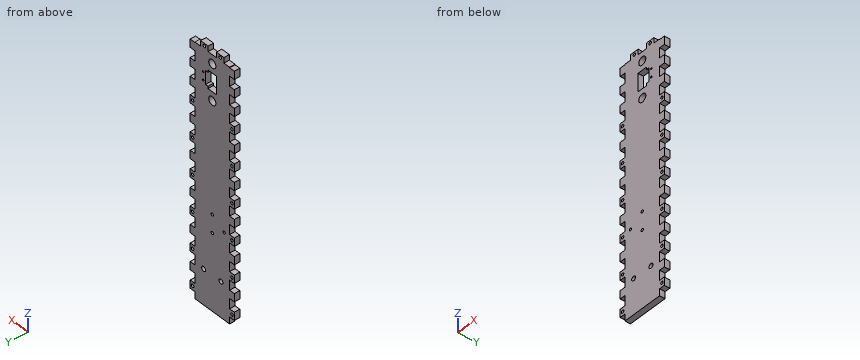
from build123d import *

# Parameters (mm, degrees)
SKETCH1_W               = 44
SKETCH1_H               = 6
BOSS_EXTRUDE1_DEPTH     = 277
SKETCH4_W               = 9
SKETCH4_H               = 6
BOSS_EXTRUDE2_DEPTH     = 6
SKETCH5_W               = 9
SKETCH5_H               = 6
BOSS_EXTRUDE3_DEPTH     = 6
SKETCH6_W               = 9.5
SKETCH6_H               = 6
BOSS_EXTRUDE4_DEPTH     = 6
SKETCH7_R               = 1.6
CUT_EXTRUDE1_DEPTH      = 286.346184868
SKETCH8_R               = 2.5
CUT_EXTRUDE2_DEPTH      = 12
SKETCH9_R               = 1.6
CUT_EXTRUDE3_DEPTH      = 12
SKETCH11_W              = 11
SKETCH11_H              = 20
SKETCH11_W_2            = 3.1
SKETCH11_H_2            = 15
SKETCH11_R              = 4.5
SKETCH11_R_2            = 1
CUT_EXTRUDE4_DEPTH      = 286.346184868
SKETCH7_2_R             = 1.6
BOSS_EXTRUDE5_DEPTH     = 6
CUT_EXTRUDE5_DEPTH      = 286.346184868
CUT_EXTRUDE5_DEPTH_BACK = 286.346184868
SKETCH12_R              = 1.5


with BuildPart() as part:
    # Sketch1 → Boss-Extrude1 (new body)
    with BuildSketch(Plane.XY):
        with Locations((-8.02006689, 7.52173913)):
            Rectangle(SKETCH1_W, SKETCH1_H)
    extrude(amount=BOSS_EXTRUDE1_DEPTH)

    # Sketch4 → Boss-Extrude2 (add)
    with BuildSketch(Plane(origin=(13.97993311, 0, 0), x_dir=(0, 0, -1), z_dir=(1, 0, 0))):
        with Locations((-272, 7.52173913)):
            Rectangle(SKETCH4_W, SKETCH4_H)
        with Locations((-252, 7.52173913)):
            Rectangle(SKETCH4_W, SKETCH4_H)
        with Locations((-232, 7.52173913)):
            Rectangle(SKETCH4_W, SKETCH4_H)
        with Locations((-212, 7.52173913)):
            Rectangle(SKETCH4_W, SKETCH4_H)
        with Locations((-192, 7.52173913)):
            Rectangle(SKETCH4_W, SKETCH4_H)
        with Locations((-172, 7.52173913)):
            Rectangle(SKETCH4_W, SKETCH4_H)
        with Locations((-152, 7.52173913)):
            Rectangle(SKETCH4_W, SKETCH4_H)
        with Locations((-132, 7.52173913)):
            Rectangle(SKETCH4_W, SKETCH4_H)
        with Locations((-112, 7.52173913)):
            Rectangle(SKETCH4_W, SKETCH4_H)
        with Locations((-92, 7.52173913)):
            Rectangle(SKETCH4_W, SKETCH4_H)
        with Locations((-72, 7.52173913)):
            Rectangle(SKETCH4_W, SKETCH4_H)
        with Locations((-52, 7.52173913)):
            Rectangle(SKETCH4_W, SKETCH4_H)
        with Locations((-32, 7.52173913)):
            Rectangle(SKETCH4_W, SKETCH4_H)
        with Locations((-12, 7.52173913)):
            Rectangle(SKETCH4_W, SKETCH4_H)
    extrude(amount=BOSS_EXTRUDE2_DEPTH)

    # Sketch5 → Boss-Extrude3 (add)
    with BuildSketch(Plane.ZY.offset(30.02006689)):
        with Locations((272, 7.52173913)):
            Rectangle(SKETCH5_W, SKETCH5_H)
        with Locations((252, 7.52173913)):
            Rectangle(SKETCH5_W, SKETCH5_H)
        with Locations((232, 7.52173913)):
            Rectangle(SKETCH5_W, SKETCH5_H)
        with Locations((212, 7.52173913)):
            Rectangle(SKETCH5_W, SKETCH5_H)
        with Locations((192, 7.52173913)):
            Rectangle(SKETCH5_W, SKETCH5_H)
        with Locations((172, 7.52173913)):
            Rectangle(SKETCH5_W, SKETCH5_H)
        with Locations((152, 7.52173913)):
            Rectangle(SKETCH5_W, SKETCH5_H)
        with Locations((132, 7.52173913)):
            Rectangle(SKETCH5_W, SKETCH5_H)
        with Locations((112, 7.52173913)):
            Rectangle(SKETCH5_W, SKETCH5_H)
        with Locations((92, 7.52173913)):
            Rectangle(SKETCH5_W, SKETCH5_H)
        with Locations((72, 7.52173913)):
            Rectangle(SKETCH5_W, SKETCH5_H)
        with Locations((52, 7.52173913)):
            Rectangle(SKETCH5_W, SKETCH5_H)
        with Locations((32, 7.52173913)):
            Rectangle(SKETCH5_W, SKETCH5_H)
        with Locations((12, 7.52173913)):
            Rectangle(SKETCH5_W, SKETCH5_H)
    extrude(amount=BOSS_EXTRUDE3_DEPTH)

    # Sketch6 → Boss-Extrude4 (add)
    with BuildSketch(Plane.XY.offset(277)):
        with Locations((-18.02006689, 7.52173913)):
            Rectangle(SKETCH6_W, SKETCH6_H)
        with Locations((1.97993311, 7.52173913)):
            Rectangle(SKETCH6_W, SKETCH6_H)
    extrude(amount=BOSS_EXTRUDE4_DEPTH)

    # Sketch7 → Cut-Extrude1 (cut, through all)
    with BuildSketch(Plane.XZ.offset(-4.52173913)):
        with Locations(Location((16.97993311, 252, 0), (0, 0, 270))):
            Circle(SKETCH7_R)
        with Locations(Location((-33.02006689, 252, 0), (0, 0, 90))):
            Circle(SKETCH7_R)
        with Locations(Location((-33.02006689, 212, 0), (0, 0, 90))):
            Circle(SKETCH7_R)
        with Locations(Location((16.97993311, 212, 0), (0, 0, 270))):
            Circle(SKETCH7_R)
        with Locations(Location((-33.02006689, 172, 0), (0, 0, 90))):
            Circle(SKETCH7_R)
        with Locations(Location((16.97993311, 172, 0), (0, 0, 270))):
            Circle(SKETCH7_R)
        with Locations(Location((-33.02006689, 132, 0), (0, 0, 90))):
            Circle(SKETCH7_R)
        with Locations(Location((16.97993311, 132, 0), (0, 0, 270))):
            Circle(SKETCH7_R)
        with Locations(Location((-33.02006689, 92, 0), (0, 0, 90))):
            Circle(SKETCH7_R)
        with Locations(Location((16.97993311, 92, 0), (0, 0, 270))):
            Circle(SKETCH7_R)
        with Locations(Location((-33.02006689, 52, 0), (0, 0, 90))):
            Circle(SKETCH7_R)
        with Locations(Location((16.97993311, 52, 0), (0, 0, 270))):
            Circle(SKETCH7_R)
        with Locations(Location((-33.02006689, 12, 0), (0, 0, 90))):
            Circle(SKETCH7_R)
        with Locations(Location((16.97993311, 12, 0), (0, 0, 270))):
            Circle(SKETCH7_R)
    extrude(amount=-CUT_EXTRUDE1_DEPTH, mode=Mode.SUBTRACT)

    # Sketch8 → Cut-Extrude2 (cut)
    with BuildSketch(Plane.XZ.offset(-4.52173913)):
        with Locations(Location((-19.02006689, 39, 0), (0, 0, 270))):
            Circle(SKETCH8_R)
        with Locations(Location((2.97993311, 39, 0), (0, 0, 270))):
            Circle(SKETCH8_R)
    extrude(amount=-CUT_EXTRUDE2_DEPTH, mode=Mode.SUBTRACT)

    # Sketch9 → Cut-Extrude3 (cut)
    with BuildSketch(Plane(origin=(0, 4.52173913, 0), x_dir=(-1, 0, 0), z_dir=(0, -1, 0))):
        with Locations(Location((18.02006689, -280, 0), (0, 0, 90))):
            Circle(SKETCH9_R)
        with Locations(Location((-1.97993311, -280, 0), (0, 0, 90))):
            Circle(SKETCH9_R)
    extrude(amount=-CUT_EXTRUDE3_DEPTH, mode=Mode.SUBTRACT)

    # Sketch11 → Cut-Extrude4 (cut, through all)
    with BuildSketch(Plane.XZ.offset(-4.52173913)):
        with Locations((-8.02006689, 247)):
            Rectangle(SKETCH11_W, SKETCH11_H)
        with Locations((-0.97006689, 247)):
            Rectangle(SKETCH11_W_2, SKETCH11_H_2)
        with Locations(Location((-8.02006689, 267, 0), (0, 0, 270))):
            Circle(SKETCH11_R)
        with Locations(Location((-8.02006689, 227, 0), (0, 0, 270))):
            Circle(SKETCH11_R)
        with Locations(Location((3.57993311, 251.5, 0), (0, 0, 270))):
            Circle(SKETCH11_R_2)
        with Locations(Location((3.57993311, 242.5, 0), (0, 0, 270))):
            Circle(SKETCH11_R_2)
    extrude(amount=-CUT_EXTRUDE4_DEPTH, mode=Mode.SUBTRACT)

    # Sketch7<2> → Boss-Extrude5 (add, through all)
    with BuildSketch(Plane.XZ.offset(-4.52173913)):
        with Locations((-33.02006689, 252)):
            Circle(SKETCH7_2_R)
        with Locations((16.97993311, 252)):
            Circle(SKETCH7_2_R)
    extrude(amount=-BOSS_EXTRUDE5_DEPTH)

    # Sketch12 → Cut-Extrude5 (cut, two sides: drawn at the far end of the back side and taken through both)
    with BuildSketch(Plane(origin=(0, 10.52173913, 0), x_dir=(1, 0, 0), z_dir=(0, 1, 0)).offset(-CUT_EXTRUDE5_DEPTH_BACK)):
        with Locations(Location((-8.02006689, -104.5, 0), (0, 0, 270))):
            Circle(SKETCH12_R)
        with Locations(Location((-8.02006689, -84.5, 0), (0, 0, 270))):
            Circle(SKETCH12_R)
        with Locations(Location((-23.02006689, -94.5, 0), (0, 0, 270))):
            Circle(SKETCH12_R)
    extrude(amount=CUT_EXTRUDE5_DEPTH + CUT_EXTRUDE5_DEPTH_BACK, mode=Mode.SUBTRACT)


solid = part.part
Build history of the part. All positions in model axes, mm. Give positions to 0.01 mm unless a question says otherwise; leave off trailing zeros. Write each loop counter-clockwise with the first axis right and the second up, starting at its lowest first coordinate (ties: lowest second). Pieces come first, ordered by that corner, then holes. Notation, with made-up numbers: (22, -26.5) - (76, -26.5) arc R13 cw to (76, -1.5) - close; hole circle Ø9 at (-16, 79.25). An arc over 180 degrees is marked (long way). Use one line per item in the form item = value. Start each with the question number.
1. Probe line 1 (X direction, y = 10.25, z = 39); line 2 (X direction, y = 6.4, z = 212); line 3 (X direction, y = 8.9, z = 280). List the from-to ranges inside material, lowest first. Write a range as [from, to].
2. Band-saw the part on B-B on z = 164.5. Write the cut outline in (x, y), plus the area to 3 significant figures.
3. Drop flat-ended pins along their axis: pin 1 Ø3 at (x, y) = (-32.5, 6) entering from -Z; pin 2 Ø3 at (y, z) = (10, 138.5) entering from -X; pin 3 Ø1 at (y, z) = (7, 125.5) entering from +X; pin 4 Ø3 at (x, z) = (16.98, 132) entering from -Y. Give the stop position or say it passes through.
4. Band-saw the part on A-A on y = 7.5. Count the separate pieces of the cut face and the enclosed holes in it, plus the area to 3 significant figures.
Conclusion:
q1.line_1 = [-30.02, -21.52], [-16.52, 0.48], [5.48, 13.98]
q1.line_2 = [-36.02, -34.62], [-31.42, 15.38], [18.58, 19.98]
q1.line_3 = [-22.77, -19.62], [-16.42, -13.27], [-2.77, 0.38], [3.58, 6.73]
q2.outline = (-30.02, 4.52) - (13.98, 4.52) - (13.98, 10.52) - (-30.02, 10.52) - close
q2.area = 264 mm²
q3.pin_1 = 7.5
q3.pin_2 = -30.02
q3.pin_3 = 13.98
q3.pin_4 = through
q4.separate_pieces = 1
q4.enclosed_holes = 24
q4.area = 13,200 mm²
